Could you check a few things on this model? Use its own coordinates, in mm. Face numbers are marked on the shaded views. A direction names the side the tool comes from. Coordinates: 2 decimals unless noted, no trailing zeros. Loops run counter-clockwise (first coordinate to the right, second up) from the corner with the lowest first, then second, coordinate; pieces in that order, holes last. Notation, with made-up numbers: (-0.5, 24) -> (38.5, 24) arc R20 ccw to (38.5, 34) -> close; hole circle Ø1 at (56, 60.25). An arc over 180 degrees is marked (long way). One line per question, with ' | ' between items.
```python
from build123d import *

# Parameters (mm, degrees)
SKETCH_1_W          = 55
SKETCH_1_H          = 25
EXTRUDE_1_DEPTH     = 3
SKETCH_2_W          = 55
SKETCH_2_H          = 3
EXTRUDE_2_DEPTH     = 35
SKETCH_3_W          = 5
SKETCH_3_H          = 3
EXTRUDE_3_DEPTH     = 22
CUT_EXTRUDE_1_REACH = 50.544
SKETCH_4_R          = 1.65
SKETCH_7_R          = 1.65
CUT_EXTRUDE_2_DEPTH = 20


with BuildPart() as part:
    # 草图1 → 凸台-拉伸1 (new body)
    with BuildSketch(Plane.XY):
        Rectangle(SKETCH_1_W, SKETCH_1_H)
    extrude(amount=EXTRUDE_1_DEPTH)

    # 草图2 → 凸台-拉伸2 (add)
    with BuildSketch(Plane.XY.offset(3)):
        with Locations((0, 11)):
            Rectangle(SKETCH_2_W, SKETCH_2_H)
    extrude(amount=EXTRUDE_2_DEPTH)

    # 草图3 → 凸台-拉伸3 (add)
    with BuildSketch(Plane.XZ.offset(-9.5)):
        with Locations((-25, 36.5)):
            Rectangle(SKETCH_3_W, SKETCH_3_H)
        with Locations((25, 36.5)):
            Rectangle(SKETCH_3_W, SKETCH_3_H)
    extrude(amount=EXTRUDE_3_DEPTH)

    # 草图4 → 切除-拉伸1 (cut, up to next)
    with BuildSketch(Plane.XY.offset(38), mode=Mode.PRIVATE) as cut_extrude_1_sk1:
        with Locations((-25, -5.5)):
            Circle(SKETCH_4_R)
    cut_extrude_1_tool1 = extrude(cut_extrude_1_sk1.sketch, amount=-CUT_EXTRUDE_1_REACH, mode=Mode.PRIVATE) & part.part
    # 草图4 → 切除-拉伸1 (cut, up to next)
    with BuildSketch(Plane.XY.offset(38), mode=Mode.PRIVATE) as cut_extrude_1_sk2:
        with Locations((-25, 4.5)):
            Circle(SKETCH_4_R)
    cut_extrude_1_tool2 = extrude(cut_extrude_1_sk2.sketch, amount=-CUT_EXTRUDE_1_REACH, mode=Mode.PRIVATE) & part.part
    # 草图4 → 切除-拉伸1 (cut, up to next)
    with BuildSketch(Plane.XY.offset(38), mode=Mode.PRIVATE) as cut_extrude_1_sk3:
        with Locations((25, 4.5)):
            Circle(SKETCH_4_R)
    cut_extrude_1_tool3 = extrude(cut_extrude_1_sk3.sketch, amount=-CUT_EXTRUDE_1_REACH, mode=Mode.PRIVATE) & part.part
    # 草图4 → 切除-拉伸1 (cut, up to next)
    with BuildSketch(Plane.XY.offset(38), mode=Mode.PRIVATE) as cut_extrude_1_sk4:
        with Locations((25, -5.5)):
            Circle(SKETCH_4_R)
    cut_extrude_1_tool4 = extrude(cut_extrude_1_sk4.sketch, amount=-CUT_EXTRUDE_1_REACH, mode=Mode.PRIVATE) & part.part
    add(cut_extrude_1_tool1.solids().sort_by_distance((-25, -5.5, 38))[0], mode=Mode.SUBTRACT)
    add(cut_extrude_1_tool2.solids().sort_by_distance((-25, 4.5, 38))[0], mode=Mode.SUBTRACT)
    add(cut_extrude_1_tool3.solids().sort_by_distance((25, 4.5, 38))[0], mode=Mode.SUBTRACT)
    add(cut_extrude_1_tool4.solids().sort_by_distance((25, -5.5, 38))[0], mode=Mode.SUBTRACT)

    # 草图7 → 切除-拉伸2 (cut)
    with BuildSketch(Plane.XY.offset(3)):
        with Locations((17.95, -0.5)):
            Circle(SKETCH_7_R)
        with Locations((10.95, 6.5)):
            Circle(SKETCH_7_R)
        with Locations((3.95, -0.5)):
            Circle(SKETCH_7_R)
        with Locations((10.95, -7.5)):
            Circle(SKETCH_7_R)
    extrude(amount=-CUT_EXTRUDE_2_DEPTH, mode=Mode.SUBTRACT)


solid = part.part
```
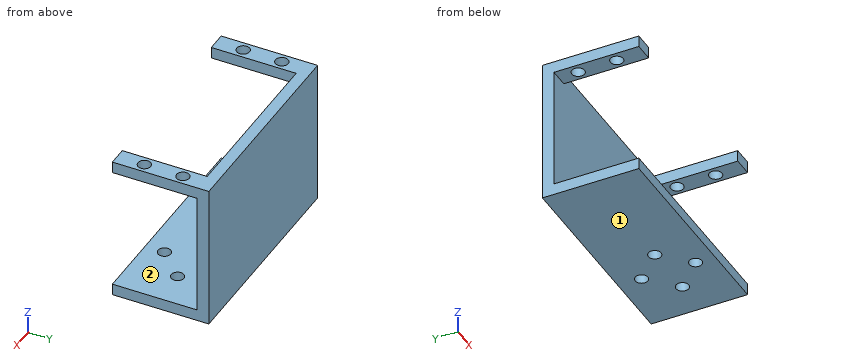
Q1. Imagine slicing it at D-D on x = 17.95. Write out the boundary of the cut face in (y, z), plus the area to 3 significant figures.
Values follow:
outline: (-12.5, 0) -> (-2.15, 0) -> (-2.15, 3) -> (-12.5, 3) -> close; (1.15, 0) -> (12.5, 0) -> (12.5, 38) -> (9.5, 38) -> (9.5, 3) -> (1.15, 3) -> close | area: 170 mm2
Q2. For the marked faces 1 and 2, which set-ups out of +Z, -Z, +X, -X, +Y, -Y let a thin tool reach every point of the face, with its end or its side?
Values follow:
face 1: -Z, +X, -X, +Y, -Y | face 2: +X, -X, -Y
Q3. For pin 1 (4 mm diameter, centred on x = 1, z = 9, fed in from -Y); pin 2 (4 mm diameter, centred on x = 10.95, y = -7.5, fed in from +Z), each with a flat end and sliding along its axis, tell me the tip position at first contact or that it passes through.
Values follow:
pin 1: stops at y = 9.5 | pin 2: stops at z = 3
Q4. Imagine slicing it at A-A on y = 2. Write out the boundary of the cut face in (x, z).
Values follow:
outline: (-27.5, 0) -> (27.5, 0) -> (27.5, 3) -> (-27.5, 3) -> close; (-27.5, 35) -> (-22.5, 35) -> (-22.5, 38) -> (-27.5, 38) -> close; (22.5, 35) -> (27.5, 35) -> (27.5, 38) -> (22.5, 38) -> close
Q5. Imagine slicing it at C-C on y = -0.5. Write out the boundary of the cut face in (x, z).
Values follow:
outline: (-27.5, 0) -> (2.3, 0) -> (2.3, 3) -> (-27.5, 3) -> close; (-27.5, 35) -> (-22.5, 35) -> (-22.5, 38) -> (-27.5, 38) -> close; (5.6, 0) -> (16.3, 0) -> (16.3, 3) -> (5.6, 3) -> close; (19.6, 0) -> (27.5, 0) -> (27.5, 3) -> (19.6, 3) -> close; (22.5, 35) -> (27.5, 35) -> (27.5, 38) -> (22.5, 38) -> close
Q6. Imagine slicing it at B-B on x = 10.95. Write out the boundary of the cut face in (y, z), plus the area to 3 significant figures.
Values follow:
outline: (-12.5, 0) -> (-9.15, 0) -> (-9.15, 3) -> (-12.5, 3) -> close; (-5.85, 0) -> (4.85, 0) -> (4.85, 3) -> (-5.85, 3) -> close; (8.15, 0) -> (12.5, 0) -> (12.5, 38) -> (9.5, 38) -> (9.5, 3) -> (8.15, 3) -> close | area: 160 mm2
Q7. Please list where these lines run through material, in increasing order: L1, parallel to Y at x = 25, z = 36.85; L2, parallel to Z at x = -4.5, y = 3.75; L3, parallel to Y at x = 2, z = 35. Write a range as [from, to].
Values follow:
L1: y = [-12.5, -7.15], [-3.85, 2.85], [6.15, 12.5] | L2: z = [0, 3] | L3: y = [9.5, 12.5]
